Source: CAD feature listing. Evaluate the final solid. Frame: model axes, mm. Face numbers are marked on the shaded views. Round coordinates to 2 decimals unless told otherwise and drop trailing zeros. Write each loop counter-clockwise with the first axis right and the second up, starting at its lowest first coordinate (ties: lowest second). Pieces come first, ordered by that corner, then holes. Notation, with made-up numbers: M 48.5,25.5 L 101.5,25.5 A21 ccw 101.5,61.5 Z; hole C -37.75,84.25 d9. An arc over 180 degrees is marked long. Answer in a Markdown table with one row per item.
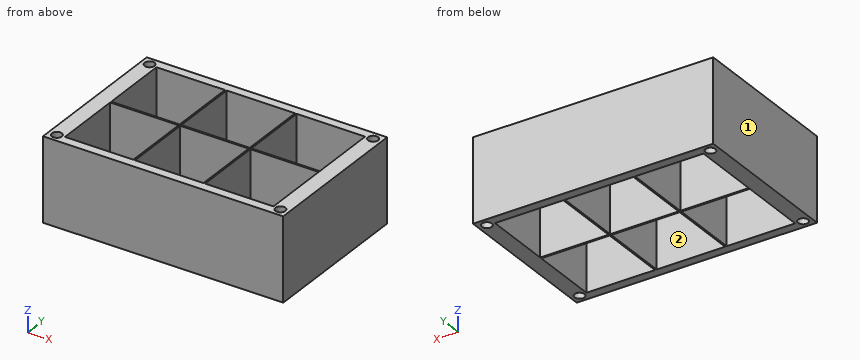
from build123d import *

# Parameters (mm, degrees)
SKETCH_1_W          = 72
SKETCH_1_H          = 47
SKETCH_1_W_2        = 20.5
SKETCH_1_H_2        = 20.5
EXTRUDE_1_DEPTH     = 25
SKETCH_2_R          = 1.5
CUT_EXTRUDE_1_DEPTH = 26


with BuildPart() as part:
    # ｽｹｯﾁ1 → ﾎﾞｽ - 押し出し1 (new body)
    with BuildSketch(Plane.XY):
        with Locations((-49.384838442, 41.173989141)):
            Rectangle(SKETCH_1_W, SKETCH_1_H)
        with Locations((-49.384838442, 30.673989141)):
            Rectangle(SKETCH_1_W_2, SKETCH_1_H_2, mode=Mode.SUBTRACT)
        with Locations((-70.384838442, 30.673989141)):
            Rectangle(SKETCH_1_W_2, SKETCH_1_H_2, mode=Mode.SUBTRACT)
        with Locations((-28.384838442, 30.673989141)):
            Rectangle(SKETCH_1_W_2, SKETCH_1_H_2, mode=Mode.SUBTRACT)
        with Locations((-49.384838442, 51.673989141)):
            Rectangle(SKETCH_1_W_2, SKETCH_1_H_2, mode=Mode.SUBTRACT)
        with Locations((-28.384838442, 51.673989141)):
            Rectangle(SKETCH_1_W_2, SKETCH_1_H_2, mode=Mode.SUBTRACT)
        with Locations((-70.384838442, 51.673989141)):
            Rectangle(SKETCH_1_W_2, SKETCH_1_H_2, mode=Mode.SUBTRACT)
    extrude(amount=EXTRUDE_1_DEPTH)

    # ｽｹｯﾁ2 → ｶｯﾄ - 押し出し1 (cut, through all)
    with BuildSketch(Plane.XY.offset(25)):
        with Locations((-15.884838442, 62.173989141)):
            Circle(SKETCH_2_R)
        with Locations((-82.884838442, 62.173989141)):
            Circle(SKETCH_2_R)
        with Locations((-82.884838442, 20.173989141)):
            Circle(SKETCH_2_R)
        with Locations((-15.884838442, 20.173989141)):
            Circle(SKETCH_2_R)
    extrude(amount=-CUT_EXTRUDE_1_DEPTH, mode=Mode.SUBTRACT)


solid = part.part
Q1. Section A-A (y = 49.5). Return loops of the section in (x, z).
Solutions:
| item | result |
|---|---|
| outline | M -85.38,0 L -80.63,0 L -80.63,25 L -85.38,25 Z; M -60.13,0 L -59.63,0 L -59.63,25 L -60.13,25 Z; M -39.13,0 L -38.63,0 L -38.63,25 L -39.13,25 Z; M -18.13,0 L -13.38,0 L -13.38,25 L -18.13,25 Z |
Q2. Contact query for a flat-ended pin moving along its axis: pin 1 Ø2.5 at (x, y) = (-82.88, 62.17) entering from -Z. Output: stop coordinate, or through.
Solutions:
| item | result |
|---|---|
| pin 1 | passes through |
Q3. Pull-direction query (Y, two-part tool) for the marked faces 1 and 2; classes: pulls with the +Y half, pulls with the -Y half, needs draft (parallel to the pull), parting line crosses it, or undercut.
Solutions:
| item | result |
|---|---|
| face 1 | needs draft |
| face 2 | undercut |
Q4. Section C-C (z = 19). State how many separate pieces and enclosed holes the cut face has, and give its area (3 significant figures).
Solutions:
| item | result |
|---|---|
| separate pieces | 1 |
| enclosed holes | 10 |
| area | 834 mm2 |
Q5. Material intervals for probe 1 along X at (y, z) = (25, 14.5); probe 2 along Y at (x, z) = (-75, 23); probe 3 along X at (y, z) = (21, 13.5), sorted ascending.
Solutions:
| item | result |
|---|---|
| probe 1 | x = -85.38 to -80.63, -60.13 to -59.63, -39.13 to -38.63, -18.13 to -13.38 |
| probe 2 | y = 17.67 to 20.42, 40.92 to 41.42, 61.92 to 64.67 |
| probe 3 | x = -85.38 to -84.14, -81.63 to -80.63, -60.13 to -59.63, -39.13 to -38.63, -18.13 to -17.14, -14.63 to -13.38 |
Q6. Section B-B (x = -54.5). Return loops of the section in (y, z), and give its area (3 significant figures).
Solutions:
| item | result |
|---|---|
| outline | M 17.67,0 L 20.42,0 L 20.42,25 L 17.67,25 Z; M 40.92,0 L 41.42,0 L 41.42,25 L 40.92,25 Z; M 61.92,0 L 64.67,0 L 64.67,25 L 61.92,25 Z |
| area | 150 mm2 |
